For this review, take the finished solid that the model builds, in its own axes (mm). A direction names the side the tool comes from. Give positions to 0.01 mm unless a question says otherwise; leave off trailing zeros. Order: outer loops, then holes, each group sorted by start corner. A loop starts at its lowest first (then second) coordinate and runs counter-clockwise, first axis right, second up. Notation, with made-up numbers: (-1, 74) - (51, 74) arc R31 ccw to (51, 107) - close; hole circle Ø10 at (65.5, 60.5). An arc over 180 degrees is marked (long way). One line per item, written item: value.
```python
from build123d import *

# Parameters (mm, degrees)
F0_R     = 330.2
F1_DEPTH = 25.4
F4_W     = 47.625
F4_H     = 47.625
F5_DEPTH = 660.4
F7_DEPTH = 47.625


with BuildPart() as f1:
    # F0 (on Top) → F1 (new body)
    with BuildSketch(Plane.XY):
        Circle(F0_R)
    extrude(amount=F1_DEPTH)

    # F2 (on Front) → F3 (revolve, cut)
    with BuildSketch(Plane.XZ):
        with BuildLine():
            Line((-317.797519, 22.86), (-317.797519, 25.4))
            Line((-317.797519, 25.4), (-330.497519, 25.4))
            Line((-330.497519, 25.4), (-330.497519, 12.7))
            ThreePointArc((-330.497519, 12.7), (-325.987211, 20.079616), (-317.797519, 22.86))
        make_face()
    revolve(axis=Axis((0, 0, -14.905058), (0, 0, -1)), mode=Mode.SUBTRACT)

    # F4 (on face) → F5 (join)
    with BuildSketch(Plane(origin=(0, 0, 0), x_dir=(1, 0, 0), z_dir=(0, 0, -1))):
        Rectangle(F4_W, F4_H)
    extrude(amount=F5_DEPTH)

    # F6 (on face) → F7 (join)
    with BuildSketch(Plane(origin=(-23.8125, 0, 0), x_dir=(0, -1, 0), z_dir=(-1, 0, 0))):
        with BuildLine():
            Line((204.1525, -584.2), (153.3525, -584.2))
            ThreePointArc((153.3525, -584.2), (98.428054, -529.940923), (23.8125, -510.110108))
            Line((23.8125, -510.110108), (23.8125, -586.310108))
            ThreePointArc((23.8125, -586.310108), (80.612019, -612.922013), (121.6025, -660.4))
            Line((121.6025, -660.4), (204.1525, -660.4))
            Line((204.1525, -660.4), (204.1525, -584.2))
        make_face()
    extrude(amount=-F7_DEPTH)


solid = f1.part
```
(1) Take a section at B-B (y = 0). Write out the cut boundary in (x, z).
Answers below:
outline: (-330.2, 0) - (-23.81, 0) - (-23.81, -660.4) - (23.81, -660.4) - (23.81, 0) - (330.2, 0) - (330.2, 13.87) arc R12.7 ccw to (317.8, 22.86) - (317.8, 25.4) - (-317.8, 25.4) - (-317.8, 22.86) arc R12.7 ccw to (-330.2, 13.87) - close
(2) Machinability: for faces 4 (the face through (0, -204.152, -623)), 5 (the face through (252.193, -193.375, 24.148)), 6 (the face through (0, -23.812, -251)), which of the approach directions +Z, -Z, +X, -X, +Y, -Y give a long, thin tool a straight path to every point of the face, cutting with its end or side? Answer none if there is none.
Answers below:
face 4: -Z, +X, -X, -Y
face 5: +Z
face 6: +X, -X, -Y
(3) Take a section at A-A (x = 0). Write out the cut boundary in (y, z).
Answers below:
outline: (-330.2, 0) - (-23.81, 0) - (-23.81, -510.11) arc R150.29 ccw to (-153.35, -584.2) - (-204.15, -584.2) - (-204.15, -660.4) - (-121.6, -660.4) arc R150.29 cw to (-23.81, -586.31) - (-23.81, -660.4) - (23.81, -660.4) - (23.81, 0) - (330.2, 0) - (330.2, 13.87) arc R12.7 ccw to (317.8, 22.86) - (317.8, 25.4) - (-317.8, 25.4) - (-317.8, 22.86) arc R12.7 ccw to (-330.2, 13.87) - close
(4) Draft analysis for pull direction Z (two halves, no side actions). For faces 1 (the face through (0, 0, -660.4)), 2 (the face through (-23.812, -22, -402)), 3 (the face through (-0.3, -99.4, -530.5)), state which applies: pulls with the +Z half, pulls with the -Z half, needs draft (parallel to the pull), parting line crosses it, or undercut.
Answers below:
face 1: pulls with the -Z half
face 2: needs draft
face 3: undercut
(5) Take a section at C-C (z = -303). Write out the cut boundary in (x, y), then the cut area to 3 significant figures.
Answers below:
outline: (-23.81, -23.81) - (23.81, -23.81) - (23.81, 23.81) - (-23.81, 23.81) - close
area: 2,270 mm^2
(6) Wall thickness on line 1 (Z direction, x = 295.5, y = 45.5); line 2 (X direction, y = 0, z = -289.5): over which ranges is each line inside the solid? List them lowest first. Write a range as from..to.
Answers below:
line 1: z = 0..25.4
line 2: x = -23.81..23.81
(7) For P1, Ø14.5, axis at x = -10, z = -412.5, coming from the +Y side; P2, Ø10, axis at x = -80, y = 146.5, coming from the -Z side; P3, Ø12, axis at y = -60, z = -507.5, coming from the +X side; P4, Ø14.5, axis at x = -3, z = -609, coming from the -Y side, all flat-tipped, find the tip position at first contact; note any pin that passes through.
Answers below:
P1: stops at y = 23.81
P2: stops at z = 0
P3: passes through
P4: stops at y = -204.15
